Work out the finished part from the listing and answer in its coordinate system (mm). A direction names the side the tool comes from. Round coordinates to 2 decimals unless told otherwise and drop trailing zeros. Write each loop counter-clockwise with the first axis right and the second up, starting at its lowest first coordinate (ties: lowest second). Pieces come first, ordered by that corner, then holes. Notation, with made-up numbers: (52.5, 56.25) -> (78.5, 56.25) arc R27 cw to (78.5, 90.25) -> close; hole circle Ø9 at (8.5, 35). An arc over 180 degrees is marked (long way). One line per question, with ' | ' between items. Start each with the question number.
Autodesk Inventor part; units mm, degrees
ref_plane "YZ Plane" through (0, 0, 0) normal (1, 0, 0) x (0, 1, 0)
ref_plane "XZ Plane" through (0, 0, 0) normal (0, 1, 0) x (-1, 0, 0)
ref_plane "XY Plane" through (0, 0, 0) normal (0, 0, 1) x (1, 0, 0)
sketch "Эскиз1" plane through (0, 0, 0) normal (0, 1, 0) x (-1, 0, 0)
  circle A0 centre (0, 0) radius 2.45
  dimension "d0" = 4.9
extrude "Выдавливание1" add sketch "Эскиз1" along normal blind 3
ref_plane "РабПлоскость2" through (0, 10, 0) normal (0, 1, 0) x (1, 0, 0)
sketch "Эскиз2" plane through (0, 10, 0) normal (0, 1, 0) x (1, 0, 0)
  circle A0 centre (0, 0) radius 10
  dimension "d4" = 20
extrude "Выдавливание2" add sketch "Эскиз2" along normal blind 1.5
loft "Лофт1" add section 1 edges at (-10, 10, 0) section 2 edges at (2.45, 3, 0)
sketch "Эскиз3" plane through (0, 0, 0) normal (0, -1, 0) x (1, 0, 0)
  circle A0 centre (0, 0) radius 2.45
  circle A1 centre (0, 0) radius 2
  dimension "d11" = 4
sketch "Эскиз4" plane through (0, 0, 0) normal (0, -1, 0) x (1, 0, 0)
  point P0 (0, 0)
extrude "Выдавливание3" cut sketch "Эскиз3" against normal blind 3 contours A1
sketch "Эскиз5" plane through (0, 11.5, 0) normal (0, 1, 0) x (1, 0, 0)
  circle A0 centre (0, 0) radius 9
  dimension "d14" = 18
extrude "Выдавливание4" cut sketch "Эскиз5" against normal blind 2
fillet "Сопряжение1" radius 2 3 edges at (-9, 9.5, 0) (0, 3, -2.45) (0, 3, 2.45)
sketch "Эскиз6" plane through (0, 9.5, 0) normal (0, 1, 0) x (1, 0, 0)
  circle A0 centre (0, 0) radius 7.2679
extrude "Выдавливание5" cut sketch "Эскиз6" against normal blind 1.8
fillet "Сопряжение2" radius 2 1 edges at (-7.2679, 7.7, 0)
sketch "Эскиз7" plane through (0, 7.7, 0) normal (0, 1, 0) x (1, 0, 0)
  circle A0 centre (0, 0) radius 5.5359
extrude "Выдавливание6" cut sketch "Эскиз7" against normal blind 1.8
fillet "Сопряжение3" radius 2 1 edges at (-5.5359, 5.9, 0)
sketch "Эскиз11" plane through (0, 5.9, 0) normal (0, 1, 0) x (1, 0, 0)
  circle A0 centre (0, 0) radius 2
extrude "Выдавливание10" cut sketch "Эскиз11" against normal blind 3.1
fillet "Сопряжение6" radius 2 1 edges at (-2, 5.9, 0)
properties part number "TubeExpander"
(1) A cutting plane is placed at B-B, the plane y = 9.75. Determine the outline of the cut face in (x, z).
(2) A cutting plane is placed at A-A, the plane y = 8.5. Determine the outline of the cut face in (x, z).
(3) The mould has two halves that part along Z. Classify faces 3 (the cylindrical face through (0, 2, -2)), 4 (the flat face through (1, 0, -2)), 5 (the cylindrical face through (-2.17, 10.74, -9.76)): +Z half, -Z half, draft (parallel to the pull), parting line (faces both ways), or undercut.
(4) For faces 1 (the cylindrical face through (0.5, 1, 2.4)), 2 (the flat face through (-9, 11.5, -2)), determine the directions among +Z, -Z, +X, -X, +Y, -Y from which every point of the face is accessible in a straight line to the end or side of a thin tool.
(5) Consider L1, parallel to X at y = 2.2, z = 0; L2, parallel to X at y = 9, z = -6.5. Determine where each line is inside the solid, lowest interval first.
(6) Given pin 1 Ø4 at (x, z) = (4, -7) entering from -Y; pin 2 Ø4 at (y, z) = (6.5, 7) entering from +X; pin 3 Ø1 at (x, z) = (-2, 4) entering from -Y; pin 4 Ø2.5 at (x, z) = (0, 0) entering from -Y, each flat-ended and moving along its own axis, determine where each tip first touches the part or whether it passes through.
Returned:
1) outline: circle Ø19.46 at (0, 0); hole circle Ø15.94 at (0, 0)
2) outline: circle Ø16.76 at (0, 0); hole circle Ø13.76 at (0, 0)
3) face 3: undercut | face 4: draft | face 5: parting line
4) face 1: -Y | face 2: +Z, -Z, +X, -X, +Y
5) L1: -2.45 to -2, 2 to 2.45 | L2: -6.11 to -2.98, 2.98 to 6.11
6) pin 1: y = 6.35 | pin 2: x = 5.44 | pin 3: y = 4.41 | pin 4: through
